```python
from build123d import *

# Parameters (mm, degrees)
SKETCH1_W               = 38.1
SKETCH1_H               = 12.7
SKETCH1_R               = 2.38125
BOSS_EXTRUDE1_DEPTH     = 12.7
CUT_EXTRUDE1_DEPTH      = 43.121134838
CUT_EXTRUDE1_DEPTH_BACK = 43.121134838
SKETCH2_R               = 2.38125
FILLET2_R               = 6.35
CHAMFER3_SIZE           = 0.396875


with BuildPart() as part:
    # Sketch1 → Boss-Extrude1 (new body)
    with BuildSketch(Plane(origin=(0, 0, 0), x_dir=(1, 0, 0), z_dir=(0, 1, 0))):
        with Locations((19.05, 6.35)):
            Rectangle(SKETCH1_W, SKETCH1_H)
        with Locations(Location((6.35, 6.35, 0), (0, 0, 270))):
            Circle(SKETCH1_R, mode=Mode.SUBTRACT)
        with Locations(Location((31.75, 6.35, 0), (0, 0, 270))):
            Circle(SKETCH1_R, mode=Mode.SUBTRACT)
    extrude(amount=BOSS_EXTRUDE1_DEPTH)

    # Sketch2 → Cut-Extrude1 (cut, two sides: drawn at the far end of the back side and taken through both)
    with BuildSketch(Plane.XY.offset(-CUT_EXTRUDE1_DEPTH_BACK)):
        with Locations((19.05, 6.35)):
            Circle(SKETCH2_R)
    extrude(amount=CUT_EXTRUDE1_DEPTH + CUT_EXTRUDE1_DEPTH_BACK, mode=Mode.SUBTRACT)

    # Fillet2
    fillet2_edges = [part.edges().sort_by_distance(p)[0] for p in [
        (0, 6.35, -12.7),
        (0, 6.35, 0),
        (38.1, 6.35, -12.7),
        (38.1, 6.35, 0),
    ]]
    fillet(fillet2_edges, radius=FILLET2_R - 0.0001)  # a hair under: the kernel refuses the full size

    # Chamfer3
    chamfer3_edges = [part.edges().sort_by_distance(p)[0] for p in [
        (6.35, 0, -8.73125),
        (6.35, 12.7, -8.73125),
        (31.75, 0, -8.73125),
        (31.75, 12.7, -8.73125),
        (16.66875, 6.35, -12.7),
        (16.66875, 6.35, 0),
        (19.05, 0, -12.7),
        (19.05, 0, 0),
        (36.24015735, 0, -1.85984265),
        (36.24015735, 0, -10.84015735),
        (1.85984265, 0, -1.85984265),
        (1.85984265, 0, -10.84015735),
        (19.05, 12.7, -12.7),
        (19.05, 12.7, 0),
        (36.24015735, 12.7, -1.85984265),
        (36.24015735, 12.7, -10.84015735),
        (1.85984265, 12.7, -1.85984265),
        (1.85984265, 12.7, -10.84015735),
    ]]
    chamfer(chamfer3_edges, length=CHAMFER3_SIZE)


solid = part.part
```
The listing builds one solid part. Answer for the finished solid, in the listing's coordinates (mm). Coordinates: 2 decimals unless noted, no trailing zeros. Loops run counter-clockwise (first coordinate to the right, second up) from the corner with the lowest first, then second, coordinate; pieces in that order, holes last. Notation, with made-up numbers: (-13.75, -39.75) -> (-8.75, -39.75) arc R17 ccw to (-8.75, -23.75) -> close; hole circle Ø4 at (12, -27.5). An arc over 180 degrees is marked (long way). Return JSON: item names as keys, results as strings. Group by question number.
(1) Determine the mould class of faces 1 (the cylindrical face through (36.19, 6.43, -1.81)), 2 (the cylindrical face through (34.11, 6.27, -6.66)), 3 (the cylindrical face through (21.32, 7.07, -6.43)) for opening direction Z: released by +Z, released by -Z, zero draft, split by the parting line, or undercut.
(2) A cutting plane is placed at A-A on x = 19.05. Write down the section's boundary in (y, z), and give its area (3 significant figures).
(3) A cutting plane is placed at B-B on y = 7. Count the separate pieces of the cut face and the enclosed holes in it, and give its area (3 significant figures).
(4) Find the intervals of material crossed by probe 1 along X at (y, z) = (3, -6.35); probe 2 along X at (y, z) = (9, -7.5); probe 3 along Y at (x, z) = (19, -2.5), in increasing order. Write a range as from..to.
(5) Given pin 1 Ø3 at (x, z) = (31.75, -6.35) entering from -Y; pin 2 Ø2 at (y, z) = (10, -11) entering from -X; pin 3 Ø1 at (y, z) = (4, -3) entering from -X, each flat-ended and moving along its own axis, determine where each tip first touches the part or whether it passes through.
The answers:
{
 "1": {"face 1": "released by +Z", "face 2": "undercut", "face 3": "zero draft"},
 "2": {"outline": "(0, -12.3) -> (0.4, -12.7) -> (3.57, -12.7) -> (3.97, -12.3) -> (3.97, -0.4) -> (3.57, 0) -> (0.4, 0) -> (0, -0.4) -> close; (8.73, -12.3) -> (9.13, -12.7) -> (12.3, -12.7) -> (12.7, -12.3) -> (12.7, -0.4) -> (12.3, 0) -> (9.13, 0) -> (8.73, -0.4) -> close", "area": "100 mm^2"},
 "3": {"separate pieces": "2", "enclosed holes": "2", "area": "355 mm^2"},
 "4": {"probe 1": "x = 0..3.97, 8.73..29.37, 34.13..38.1", "probe 2": "x = 0.1..4.26, 8.44..29.66, 33.84..38", "probe 3": "y = 0..3.97, 8.73..12.7"},
 "5": {"pin 1": "passes through", "pin 2": "stops at x = 1.15", "pin 3": "stops at x = 0.68"}
}
